```python
from build123d import *

# Parameters (mm, degrees)
SKETCH1_R           = 123
BOSS_EXTRUDE1_DEPTH = 6.35
SKETCH2_R           = 30.1625
CUT_EXTRUDE1_DEPTH  = 175.064133296
CUT_EXTRUDE2_REACH  = 176.064
SKETCH3_R           = 4.7625


with BuildPart() as part:
    # Sketch1 → Boss-Extrude1 (new body)
    with BuildSketch(Plane(origin=(0, 0, 0), x_dir=(1, 0, 0), z_dir=(0, 1, 0))):
        with Locations(Location((0, 0, 0), (0, 0, 270))):
            Circle(SKETCH1_R)
    extrude(amount=BOSS_EXTRUDE1_DEPTH)

    # Sketch2 → Cut-Extrude1 (cut, through all)
    with BuildSketch(Plane(origin=(0, 6.35, 0), x_dir=(1, 0, 0), z_dir=(0, 1, 0))):
        with Locations(Location((0, 0, 0), (0, 0, 270))):
            Circle(SKETCH2_R)
        with Locations(Location((-82.55, 0, 0), (0, 0, 270))):
            Circle(SKETCH2_R)
    extrude(amount=-CUT_EXTRUDE1_DEPTH, mode=Mode.SUBTRACT)

    # Sketch3 → Cut-Extrude2 (cut, up to next)
    with BuildSketch(Plane(origin=(0, 6.35, 0), x_dir=(1, 0, 0), z_dir=(0, 1, 0)), mode=Mode.PRIVATE) as cut_extrude2_sk1:
        with Locations(Location((58.371664787, -58.371664787, 0), (0, 0, 270))):
            Circle(SKETCH3_R)
    cut_extrude2_tool1 = extrude(cut_extrude2_sk1.sketch, amount=-CUT_EXTRUDE2_REACH, mode=Mode.PRIVATE) & part.part
    add(cut_extrude2_tool1.solids().sort_by_distance((58.371665, 6.35, 58.371665))[0], mode=Mode.SUBTRACT)


solid = part.part
```
Verification items for the finished model (mm, model axes). Coordinates: 2 decimals unless noted, no trailing zeros. Loops run counter-clockwise (first coordinate to the right, second up) from the corner with the lowest first, then second, coordinate; pieces in that order, holes last. Notation, with made-up numbers: (11.25, 41) -> (49.25, 41) arc R27 cw to (49.25, 76) -> close; hole circle Ø7 at (75, -21.5). An arc over 180 degrees is marked (long way). Answer in a Markdown table with one row per item. Add a question column.
1. Section check D-D, the plane z = -73. Enter the section's corners in (x, y), then the cut area to 3 significant figures.
2. Section check B-B, the plane x = 0. Enter the section's corners in (y, z).
3. Depth check by flat-ended pin: P1, Ø1, axis at x = 38.5, y = 4, coming from the -Z side; P2, Ø2, axis at y = 4, z = -68.5, coming from the -X side. Enter the tip coordinate at first touch or a pass-through.
4. Material ranges on probe 1 along X at (y, z) = (4, 0); probe 2 along X at (y, z) = (4.75, -11); probe 3 along Z at (x, y) = (58.5, 5.75), recorded low to high. Write a range as [from, to].
5. Section check A-A, the plane z = 0. Enter the section's corners in (x, y).
6. Draft check along X on faces 1 (the face through (58.581, 3.219, 53.614)), 2 (the face through (29, 0, 26)), 3 (the face through (1.326, 3.219, -30.133)), 4 (the face through (121.953, 3.131, -16.012)). Enter one of: +X half, -X half, draft (parallel to the pull), parting line (faces both ways), or undercut.
7. Section check C-C, the plane x = -82.55. Enter the section's corners in (y, z), then the cut area to 3 significant figures.
Derived:
| question | item | result |
|---|---|---|
| 1 | outline | (-98.99, 0) -> (98.99, 0) -> (98.99, 6.35) -> (-98.99, 6.35) -> close |
| 1 | area | 1,260 mm² |
| 2 | outline | (0, -123) -> (6.35, -123) -> (6.35, -30.16) -> (0, -30.16) -> close; (0, 30.16) -> (6.35, 30.16) -> (6.35, 123) -> (0, 123) -> close |
| 3 | P1 | stops at z = -116.98 |
| 3 | P2 | stops at x = -102.82 |
| 4 | probe 1 | x = [-123, -112.71], [-52.39, -30.16], [30.16, 123] |
| 4 | probe 2 | x = [-122.51, -110.64], [-54.46, -28.09], [28.09, 122.51] |
| 4 | probe 3 | z = [-108.2, 53.61], [63.13, 108.2] |
| 5 | outline | (-123, 0) -> (-112.71, 0) -> (-112.71, 6.35) -> (-123, 6.35) -> close; (-52.39, 0) -> (-30.16, 0) -> (-30.16, 6.35) -> (-52.39, 6.35) -> close; (30.16, 0) -> (123, 0) -> (123, 6.35) -> (30.16, 6.35) -> close |
| 6 | face 1 | undercut |
| 6 | face 2 | draft |
| 6 | face 3 | undercut |
| 6 | face 4 | parting line |
| 7 | outline | (0, -91.18) -> (6.35, -91.18) -> (6.35, -30.16) -> (0, -30.16) -> close; (0, 30.16) -> (6.35, 30.16) -> (6.35, 91.18) -> (0, 91.18) -> close |
| 7 | area | 775 mm² |
